```python
from build123d import *

# Parameters (mm, degrees)
SKETCH1_R               = 3
BOSS_EXTRUDE1_DEPTH     = 8
SKETCH2_R               = 5
BOSS_EXTRUDE2_DEPTH     = 5
CUT_EXTRUDE1_DEPTH      = 11.677078252
CUT_EXTRUDE1_DEPTH_BACK = 11.677078252
SKETCH3_R               = 1
CHAMFER1_SIZE           = 1
CHAMFER1_SIZE2          = 2.355852366
CHAMFER2_SIZE           = 0.5
CHAMFER2_SIZE2          = 1.177926183


with BuildPart() as part:
    # Sketch1 → Boss-Extrude1 (new body)
    with BuildSketch(Plane(origin=(0, 0, 0), x_dir=(1, 0, 0), z_dir=(0, 1, 0))):
        with Locations(Location((0, 0, 0), (0, 0, 270))):
            Circle(SKETCH1_R)
    extrude(amount=BOSS_EXTRUDE1_DEPTH)

    # Sketch2 → Boss-Extrude2 (add)
    with BuildSketch(Plane.XZ):
        with Locations(Location((0, 0, 0), (0, 0, 270))):
            Circle(SKETCH2_R)
    extrude(amount=BOSS_EXTRUDE2_DEPTH)

    # Sketch3 → Cut-Extrude1 (cut, two sides: drawn at the far end of the back side and taken through both)
    with BuildSketch(Plane.XY.offset(-CUT_EXTRUDE1_DEPTH_BACK)):
        with Locations(Location((0, -2.5, 0), (0, 0, 270))):
            Circle(SKETCH3_R)
    extrude(amount=CUT_EXTRUDE1_DEPTH + CUT_EXTRUDE1_DEPTH_BACK, mode=Mode.SUBTRACT)

    # Chamfer1
    chamfer1_edges = [part.edges().sort_by_distance(p)[0] for p in [
        (0, -5, 5),
    ]]
    chamfer1_side = [part.faces().sort_by_distance(p)[0] for p in [
        (0, -2.5, 5),
    ]]
    chamfer(chamfer1_edges, length=CHAMFER1_SIZE, length2=CHAMFER1_SIZE2, reference=chamfer1_side[0])

    # Chamfer2
    chamfer2_edges = [part.edges().sort_by_distance(p)[0] for p in [
        (0, 8, -3),
    ]]
    chamfer2_side = [part.faces().sort_by_distance(p)[0] for p in [
        (0, 4, -3),
    ]]
    chamfer(chamfer2_edges, length=CHAMFER2_SIZE, length2=CHAMFER2_SIZE2, reference=chamfer2_side[0])


solid = part.part
```
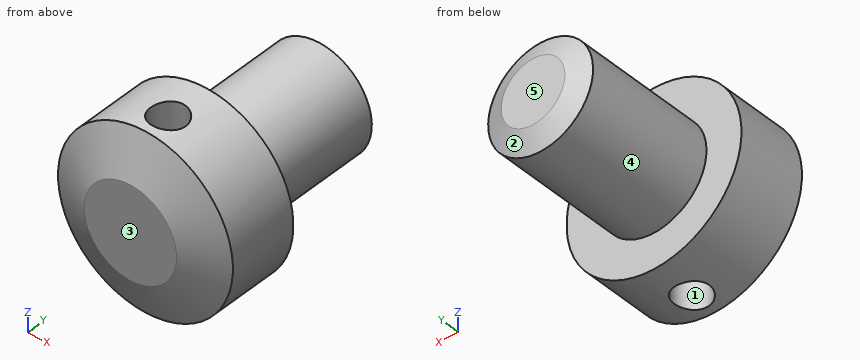
Work out the finished part from the listing and answer in its coordinate system (mm). Face numbers are marked on the shaded views. A direction names the side the tool comes from. Give positions to 0.01 mm unless a question says otherwise; leave off trailing zeros. Write each loop counter-clockwise with the first axis right and the second up, starting at its lowest first coordinate (ties: lowest second). Pieces come first, ordered by that corner, then holes.
(1) Which of the six approach directions +Z, -Z, +X, -X, +Y, -Y give full straight-line access (tool end or side, diameter ignored) to the marked faces 4 and 5?
Final values:
face 4: +Y
face 5: +Z, -Z, +X, -X, +Y
(2) The part is cut by section C-C on y = -1.75. Write down the section's boundary in (x, z).
Final values:
outline: (-0.66, -4.96) - (-0.66, 4.96) arc R5 ccw to start; (0.66, -4.96) arc R5 ccw to (0.66, 4.96) - close
(3) The mould has two halves that part along Y. Classify the marked faces 1, 2 and 3: pulls with the +Y half, pulls with the -Y half, needs draft (parallel to the pull), parting line crosses it, or undercut.
Final values:
face 1: undercut
face 2: pulls with the +Y half
face 3: pulls with the -Y half
(4) The part is cut by section D-D on y = 2.25. Write down the section's boundary in (x, z).
Final values:
outline: circle Ø6 at (0, 0)
(5) The part is cut by section A-A on x = 0. Write down the section's boundary in (y, z).
Final values:
outline: (-5, -2.64) - (-4, -5) - (-3.5, -5) - (-3.5, 5) - (-4, 5) - (-5, 2.64) - close; (-1.5, -5) - (0, -5) - (0, -3) - (7.5, -3) - (8, -1.82) - (8, 1.82) - (7.5, 3) - (0, 3) - (0, 5) - (-1.5, 5) - close
(6) Straight lines are drawn through the part: line 1 (Y direction, x = 0, z = -0.75); line 2 (X direction, y = -2.5, z = -0.25); line 3 (X direction, y = -3.25, z = -3.25). For each, find the intervals that lie inside material, in ascending order.
Final values:
line 1: y = -5 to -3.5, -1.5 to 8
line 2: x = -4.99 to -1, 1 to 4.99
line 3: x = -3.8 to -0.66, 0.66 to 3.8
(7) The part is cut by section B-B on z = 0. Write down the section's boundary in (x, y), plus the area to 3 significant figures.
Final values:
outline: (-5, -4) - (-2.64, -5) - (2.64, -5) - (5, -4) - (5, 0) - (3, 0) - (3, 7.5) - (1.82, 8) - (-1.82, 8) - (-3, 7.5) - (-3, 0) - (-5, 0) - close; hole circle Ø2 at (0, -2.5)
area: 91.9 mm2
(8) Flat-ended cylindrical pins translate along their axes: pin 1 Ø5 at (y, z) = (4.5, 2) entering from +X; pin 2 Ø2 at (y, z) = (-1.5, 4) entering from +X; pin 3 Ø1 at (y, z) = (3.5, 3) entering from +X. Find the tip coordinate at first contact, or state that the pin passes through.
Final values:
pin 1: stops at x = 3
pin 2: stops at x = 4
pin 3: stops at x = 1.66
